The listing builds one solid part. Answer for the finished solid, in the listing's coordinates (mm). Face numbers are marked on the shaded views. A direction names the side the tool comes from. Coordinates: 2 decimals unless noted, no trailing zeros. Order: outer loops, then holes, each group sorted by start corner. A loop starts at its lowest first (then second) coordinate and runs counter-clockwise, first axis right, second up.
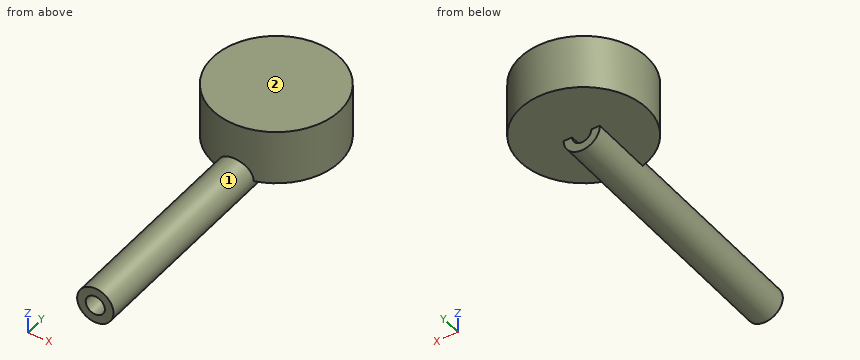
```python
from build123d import *

# Parameters (mm, degrees)
F0_R     = 33.6790507012
F0_R_2   = 17.8010861737
F1_DEPTH = 508
F2_R     = 118.1427595492
F3_DEPTH = 101.6


# Not quite as in the source:
# - the program builds the solid bodies; features that only make, move or delete a surface that nothing else refers to are left out


with BuildPart() as f1:
    # F0 (on Front) → F1 (new body)
    with BuildSketch(Plane.XZ):
        Circle(F0_R)
        Circle(F0_R_2, mode=Mode.SUBTRACT)
    extrude(amount=F1_DEPTH)

    # F2 (on Top) → F3 (join)
    with BuildSketch(Plane.XY):
        with Locations((0, -5.3212568164)):
            Circle(F2_R)
    extrude(amount=F3_DEPTH)


solid = f1.part
```
(1) Each of these flat-tipped pins is pushed along its axis until it touches: pin 1 Ø1 at (x, z) = (46, 20) entering from +Y; pin 2 Ø3 at (x, y) = (5.5, -294.5) entering from -Z; pin 3 Ø10 at (x, y) = (16, -421.5) entering from +Z. Where does it stop, or does it pass through?
(2) Find section B-B (y = -228.5). Write down the section's boundary in (x, z).
(3) Find section C-C (z = 69.5). Write down the section's boundary in (x, y), and give its area (3 significant figures).
(4) Find section A-A (x = 0). Write down the section's boundary in (y, z), and give its area (3 significant figures).
(5) For the marked faces 1 and 2, determine the directions among +Z, -Z, +X, -X, +Y, -Y from which every point of the face is accessible in a straight line to the end or side of a thin tool.
(6) Consider line 1 (Z direction, x = 0, y = -258); line 2 (Z direction, x = 102, y = -29.5). Determine where each line is inside the solid, lowest interval first.
(7) Find section D-D (x = -79). Write down the section's boundary in (y, z).
Findings below:
1. pin 1: stops at y = 103.71
1. pin 2: stops at z = -33.44
1. pin 3: stops at z = 31.83
2. outline: circle Ø67.36 at (0, 0); hole circle Ø35.6 at (0, 0)
3. outline: circle Ø236.29 at (0, -5.32)
3. area: 43,800 mm2
4. outline: (-508, -33.68) - (0, -33.68) - (0, -17.8) - (-508, -17.8) - close; (-508, 17.8) - (-123.46, 17.8) - (-123.46, 0) - (112.82, 0) - (112.82, 101.6) - (-123.46, 101.6) - (-123.46, 33.68) - (-508, 33.68) - close
4. area: 38,200 mm2
5. face 1: -Y
5. face 2: +Z, +X, -X, +Y, -Y
6. line 1: z = -33.68 to -17.8, 17.8 to 33.68
6. line 2: z = 0 to 101.6
7. outline: (-93.17, 0) - (82.52, 0) - (82.52, 101.6) - (-93.17, 101.6) - close
